```python
from build123d import *

# Parameters (mm, degrees)
F0_W     = 20
F0_H     = 10
F1_DEPTH = 13
F3_DEPTH = 4.3
F4_W     = 5
F4_H     = 6.5
F5_DEPTH = 15.8


with BuildPart() as f1:
    # F0 (on Top) → F1 (new body)
    with BuildSketch(Plane.XY):
        with Locations((10, 5)):
            Rectangle(F0_W, F0_H)
    extrude(amount=F1_DEPTH)

    # F2 (on face) → F3 (cut)
    with BuildSketch(Plane.YZ.offset(20)):
        Polygon((0, 13), (0, 0), (10, 13), align=None)
    extrude(amount=-F3_DEPTH, mode=Mode.SUBTRACT)

    # F4 (on face) → F5 (cut)
    with BuildSketch(Plane(origin=(0, 0, 0), x_dir=(0, -1, 0), z_dir=(-1, 0, 0))):
        with Locations((-2.5, 9.75)):
            Rectangle(F4_W, F4_H)
    extrude(amount=-F5_DEPTH, mode=Mode.SUBTRACT)


solid = f1.part
```
For this review, take the finished solid that the model builds, in its own axes (mm). A direction names the side the tool comes from. Round coordinates to 2 decimals unless told otherwise and drop trailing zeros. Order: outer loops, then holes, each group sorted by start corner. A loop starts at its lowest first (then second) coordinate and runs counter-clockwise, first axis right, second up. Notation, with made-up numbers: (-29, 12.25) -> (-18, 12.25) arc R5 cw to (-18, 18.25) -> close; hole circle Ø11 at (55, -20). An arc over 180 degrees is marked (long way). Use a Markdown table: item, result.
Item 1: Take a section at A-A (z = 3.25). State the section outline as (x, y) points.
Resolved:
| item | result |
|---|---|
| outline | (0, 0) -> (15.7, 0) -> (15.7, 2.5) -> (20, 2.5) -> (20, 10) -> (0, 10) -> close |
Item 2: For line 1 along Y through (x, z) = (1.75, 8.25); line 2 along X through (y, z) = (0.75, 5.5); line 3 along Z through (x, y) = (15.25, 1.5), list the stretches that pass through material, from the lowest coordinate up. Write a range as [from, to].
Resolved:
| item | result |
|---|---|
| line 1 | y = [5, 10] |
| line 2 | x = [0, 15.7] |
| line 3 | z = [0, 6.5] |
Item 3: Take a section at B-B (y = 4). State the section outline as (x, z) points, plus the area to 3 significant figures.
Resolved:
| item | result |
|---|---|
| outline | (0, 0) -> (20, 0) -> (20, 5.2) -> (15.7, 5.2) -> (15.7, 6.5) -> (0, 6.5) -> close |
| area | 124 mm² |
Item 4: For pin 1 (2 mm diameter, centred on x = 18, z = 3, fed in from -Y); pin 2 (2 mm diameter, centred on x = 9.5, z = 8, fed in from -Y); pin 3 (1.5 mm diameter, centred on x = 9, y = 2.5, fed in from +Z); pin 4 (4 mm diameter, centred on y = 2, z = 9.5, fed in from -X), all flat-tipped, find the tip position at first contact; note any pin that passes through.
Resolved:
| item | result |
|---|---|
| pin 1 | stops at y = 1.54 |
| pin 2 | stops at y = 5 |
| pin 3 | stops at z = 6.5 |
| pin 4 | passes through |
Item 5: Machinability: for faces 1 (the flat face through (17.88, 4.93, 6.41)), 2 (the flat face through (20, 7, 4)), 3 (the flat face through (8, 5, 10)), which of the approach directions +Z, -Z, +X, -X, +Y, -Y give a long, thin tool a straight path to every point of the face, cutting with its end or side? Answer none if there is none.
Resolved:
| item | result |
|---|---|
| face 1 | +Z, +X, -Y |
| face 2 | +Z, -Z, +X, +Y, -Y |
| face 3 | +Z, +X, -X, -Y |
Item 6: Take a section at C-C (x = 18.5). State the section outline as (y, z) points, plus the area to 3 significant figures.
Resolved:
| item | result |
|---|---|
| outline | (0, 0) -> (10, 0) -> (10, 13) -> close |
| area | 65.0 mm² |
